Verification items for the finished model (mm, model axes). A direction names the side the tool comes from. Give positions to 0.01 mm unless a question says otherwise; leave off trailing zeros. Write each loop counter-clockwise with the first axis right and the second up, starting at its lowest first coordinate (ties: lowest second). Pieces come first, ordered by that corner, then holes.
Autodesk Inventor part; units mm, degrees
ref_plane "YZ Plane" through (0, 0, 0) normal (1, 0, 0) x (0, 1, 0)
ref_plane "XZ Plane" through (0, 0, 0) normal (0, 1, 0) x (-1, 0, 0)
ref_plane "XY Plane" through (0, 0, 0) normal (0, 0, 1) x (1, 0, 0)
sketch "Sketch1" plane through (0, 0, 0) normal (0, 1, 0) x (-1, 0, 0)
  line L0 (20, 2) -> (-20, 2)
  line L1 (-20, 2) -> (-20, -2)
  line L2 (-20, -2) -> (20, -2)
  line L3 (20, -2) -> (20, 2)
  line L4 (20, 2) -> (-20, -2) construction
  line L5 (-20, 2) -> (20, -2) construction
  point P0 (0, 0)
  dimension "d0" = 40
  dimension "d1" = 4
extrude "Extrusion1" add sketch "Sketch1" along normal blind 84
sketch "Sketch2" plane through (0, 84, 0) normal (0, 1, 0) x (1, 0, 0)
  line L0 (20, 2) -> (-20, 2)
  line L1 (20, -2) -> (20, 2)
  line L2 (20, 2) -> (-20, 2)
  line L3 (-20, 2) -> (-20, -2)
  line L4 (-20, -2) -> (20, -2)
  point P0 (0, 0)
extrude "Extrusion2" add sketch "Sketch2" along normal blind 14
sketch "Sketch3" plane through (-20, 0, 2) normal (0, 0, 1) x (1, 0, 0)
  line L0 (0, 98) -> (40, 98)
  line L1 (20, 98) -> (20, 0)
  line L2 (40, 0) -> (0, 0)
  point P0 (5, 94.45)
  point P1 (35, 94.45)
  dimension "d6" = 3.55
  dimension "d7" = 30
hole "Hole1" at (-15, 94.45, 2) at (15, 94.45, 2) direction (0, 0, -1) diameter 3.1 depth 4
sketch "Sketch4" plane through (-20, 0, 2) normal (0, 0, 1) x (1, 0, 0)
  line L0 (4, 85.45) -> (36, 85.45)
  circle A0 centre (5, 94.45) radius 1.55
  circle A1 centre (35, 94.45) radius 1.55
  line L1 (0, 0) -> (40, 0)
  line L2 (40, 0) -> (40, 98)
  line L3 (0, 98) -> (40, 98)
  line L4 (0, 0) -> (0, 98)
  line L5 (40, 0) -> (40, 98)
  line L6 (4, 85.45) -> (36, 85.45)
  line L7 (36, 85.45) -> (36, 87.4)
  line L8 (36, 87.4) -> (4, 87.4)
  line L9 (4, 87.4) -> (4, 85.45)
  line L10 (0, 98) -> (40, 98)
  point P0 (20, 0)
  point P1 (20, 98)
  point P2 (20, 85.45)
  point P3 (0, 87.4)
  point P4 (40, 87.4)
  point P5 (37.1403, 85.45)
  point P6 (20, 98)
  dimension "d16" = 1.95
  dimension "d33" = 12.55
  dimension "d44" = 4
extrude "IndicatorBar" cut sketch "Sketch4" against normal blind 1 contours L9 L8 L7 L0
sketch "Sketch6" plane through (-20, 0, 2) normal (0, 0, 1) x (1, 0, 0)
  line L0 (40, 0) -> (0, 0)
  line L1 (0, 0) -> (40, 0)
  line L2 (40, 0) -> (40, -26)
  line L3 (40, -26) -> (0, -26)
  line L4 (0, -26) -> (0, 0)
  line L5 (40, 0) -> (40, 98)
  line L6 (20, -4) -> (24, -4)
  line L7 (24, -4) -> (24, -8)
  line L8 (24, -8) -> (20, -8)
  line L9 (20, -8) -> (20, -4)
  line L10 (32, -8) -> (36, -8)
  line L11 (36, -8) -> (36, -4)
  line L12 (36, -4) -> (32, -4)
  line L13 (32, -4) -> (32, -8)
  line L14 (4, -18) -> (8, -18)
  line L15 (8, -18) -> (8, -22)
  line L16 (8, -22) -> (4, -22)
  line L17 (4, -22) -> (4, -18)
  line L18 (16, -22) -> (20, -22)
  line L19 (20, -22) -> (20, -18)
  line L20 (20, -18) -> (16, -18)
  line L21 (16, -18) -> (16, -22)
  circle A0 centre (12, -20) radius 1.5
  line L22 (8, -18) -> (16, -22) construction
  line L23 (20, -8) -> (24, -8)
  line L24 (24, -8) -> (24, -12)
  line L25 (24, -12) -> (20, -12)
  line L26 (20, -12) -> (20, -8)
  line L27 (32, -8) -> (36, -8)
  line L28 (36, -8) -> (36, -12)
  line L29 (36, -12) -> (32, -12)
  line L30 (32, -12) -> (32, -8)
  line L31 (24, -4) -> (32, -12) construction
  circle A1 centre (28, -8) radius 1.5
  point P0 (20, 0)
  point P1 (40, 85.45)
  point P2 (36, -6)
  point P3 (8, -20)
  point P4 (6, -22)
  point P5 (4, -20)
  point P6 (20, -4)
  point P7 (20, -12)
  point P8 (18, -18)
  point P9 (32, -10)
  dimension "d24" = 4
  dimension "d25" = 4
  dimension "d26" = 4
  dimension "d28" = 4
  dimension "d29" = 4
  dimension "d30" = 4
  dimension "d34" = 4
  dimension "d35" = 4
  dimension "d36" = 3
  dimension "d37" = 10
  dimension "d38" = 4
  dimension "d39" = 4
  dimension "d40" = 4
  dimension "d41" = 4
  dimension "d43" = 3
extrude "UnderCar" add sketch "Sketch6" against normal blind 4
properties part number "Door_V2" material "MDF Medium Density Fiberboard"
Item 1: Set-up check for faces 1 (the face through (16, -8, 0)), 2 (the face through (0, 98, 0)): record each of +Z, -Z, +X, -X, +Y, -Y from which the full face is reachable in a straight line by a thin tool's end or side.
Answer key:
face 1: +Z, -Z
face 2: +Z, -Z, +X, -X, +Y
Item 2: Release check for a two-part mould opening along Y. For faces 3 (the face through (14.534, 92.972, -0.028)), 4 (the face through (0, 37, -2)), 5 (the face through (0, -26, 0)) record: released by +Y, released by -Y, zero draft, split by the parting line, or undercut.
Answer key:
face 3: undercut
face 4: zero draft
face 5: released by -Y
Item 3: Depth check by flat-ended pin: pin 1 (2.5 mm diameter, centred on x = 8, y = -8, fed in from -Z). Enter the tip coordinate at first touch or a pass-through.
Answer key:
pin 1: passes through
Item 4: Scan lines: line 1 along Y through (x, z) = (8, 1.15); line 2 along X through (y, z) = (-4.5, 1.35); line 3 along X through (y, z) = (94.45, 0.7). Record each from-to range of solid material in increasing order.
Answer key:
line 1: y = -26 to -9.5, -6.5 to 85.45, 87.4 to 98
line 2: x = -20 to 0, 4 to 12, 16 to 20
line 3: x = -20 to -16.55, -13.45 to 13.45, 16.55 to 20
Item 5: Sectioned sample at C-C on z = -1.25. State how many separate pieces and enclosed holes the cut face has, then the cut area to 3 significant figures.
Answer key:
separate pieces: 1
enclosed holes: 8
area: 4,830 mm2
Item 6: Sectioned sample at B-B on x = -8. Record the cut outline in (y, z), then the cut area to 3 significant figures.
Answer key:
outline: (-26, -2) - (-21.5, -2) - (-21.5, 2) - (-26, 2) - close; (-18.5, -2) - (98, -2) - (98, 2) - (87.4, 2) - (87.4, 1) - (85.45, 1) - (85.45, 2) - (-18.5, 2) - close
area: 482 mm2
Item 7: Sectioned sample at A-A on y = -8. Record the cut outline in (x, z), then the cut area to 3 significant figures.
Answer key:
outline: (-20, -2) - (0, -2) - (0, 2) - (-20, 2) - close; (4, -2) - (6.5, -2) - (6.5, 2) - (4, 2) - close; (9.5, -2) - (12, -2) - (12, 2) - (9.5, 2) - close; (16, -2) - (20, -2) - (20, 2) - (16, 2) - close
area: 116 mm2
